Part print with two shaded views. Sizes in mm from the minimum x, y, z corner. Give positions to 0.01 mm unless a question says otherwise; leave off trailing zeros. Write each loop counter-clockwise with the first axis right and the second up, starting at its lowest first coordinate (ties: lowest second). Pieces come first, ordered by that corner, then holes. Notation, with made-up numbers: (51.25, 59) - (95.25, 59) arc R15 ccw to (95.25, 85) - close; hole circle Ø5 at (73, 6). An arc over 180 degrees is marked (long way). One line per item, written item: value. Start each with the question number.
(1) Probe L1, parallel to Y at x = 50.8, z = 2.3; L2, parallel to Y at x = 83.82, z = 3.25; L3, parallel to Y at x = 86.5, z = 2.25. List the from-to ranges inside material, lowest first.
(2) Cut at B-B, the plane x = 50.8. List the corners of the cut face in (y, z) (1 decimal).
(3) Drop a flat-ended pin along its axis: P1, Ø7.5, axis at x = 50.8, y = 10.16, coming from the +Z side. Give the stop position or say it passes through.
(4) Cut at D-D, the plane x = 83.82. List the corners of the cut face in (y, z) (1 decimal), and give its area (3 significant figures).
(5) Cut at C-C, the plane z = 2.15. List the corners of the cut face in (x, y), and give its area (4 significant figures).
(6) Cut at A-A, the plane y = 60.96. List the corners of the cut face in (x, z) (1 decimal).
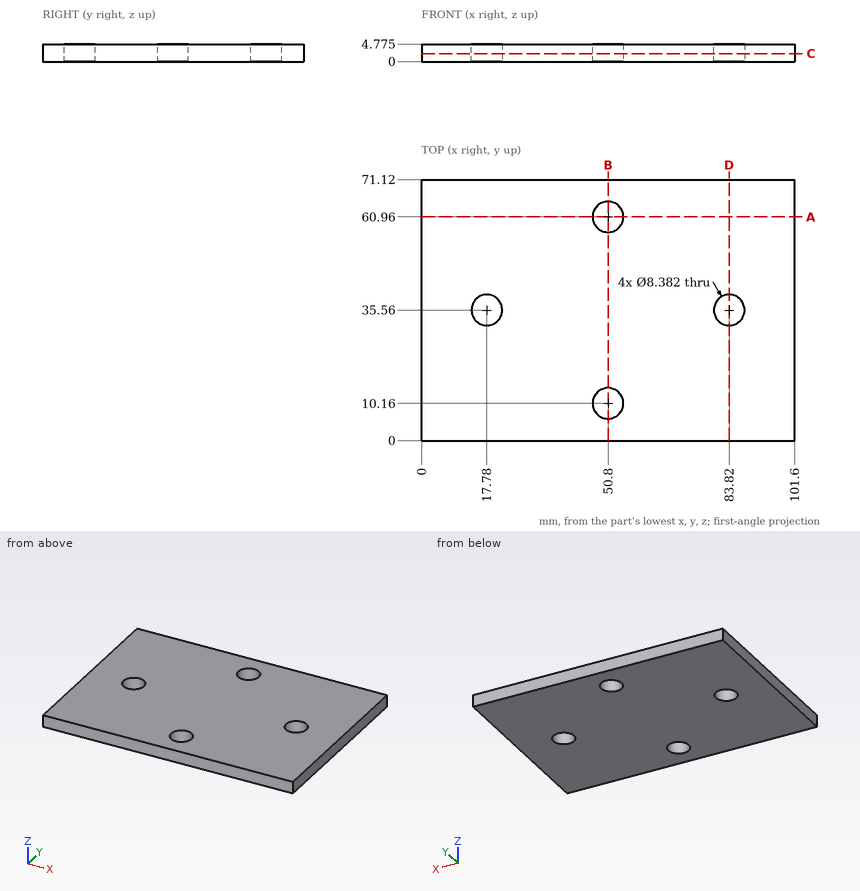
Answers follow:
1. L1: y = 0 to 5.97, 14.35 to 56.77, 65.15 to 71.12
1. L2: y = 0 to 31.37, 39.75 to 71.12
1. L3: y = 0 to 32.34, 38.78 to 71.12
2. outline: (0, 0) - (6, 0) - (6, 4.8) - (0, 4.8) - close; (14.4, 0) - (56.8, 0) - (56.8, 4.8) - (14.4, 4.8) - close; (65.2, 0) - (71.1, 0) - (71.1, 4.8) - (65.2, 4.8) - close
3. P1: passes through
4. outline: (0, 0) - (31.4, 0) - (31.4, 4.8) - (0, 4.8) - close; (39.8, 0) - (71.1, 0) - (71.1, 4.8) - (39.8, 4.8) - close
4. area: 300 mm²
5. outline: (0, 0) - (101.6, 0) - (101.6, 71.12) - (0, 71.12) - close; hole circle Ø8.38 at (17.78, 35.56); hole circle Ø8.38 at (50.8, 10.16); hole circle Ø8.38 at (50.8, 60.96); hole circle Ø8.38 at (83.82, 35.56)
5. area: 7,005 mm²
6. outline: (0, 0) - (46.6, 0) - (46.6, 4.8) - (0, 4.8) - close; (55, 0) - (101.6, 0) - (101.6, 4.8) - (55, 4.8) - close
